Build history of the part. All positions in model axes, mm. Coordinates: 2 decimals unless noted, no trailing zeros. Loops run counter-clockwise (first coordinate to the right, second up) from the corner with the lowest first, then second, coordinate; pieces in that order, holes last.
Item 1: Cut at B-B (z = -2). List the corners of the cut face in (x, y).
Item 2: Cut at A-A (y = -52). List the corners of the cut face in (x, z), and give its area (3 significant figures).
Item 3: Drill centre lines: line 1 along Z through (x, y) = (-51.5, -38); line 2 along Y through (x, z) = (-58, 82); line 3 along Y through (x, z) = (-23, 8.5). Where is each one in solid material? Low to high.
Item 4: Flat gauge pins, fed straight in: pin 1 (2 mm diameter, centred on y = 3.5, z = 7.5, fed in from -X); pin 2 (3 mm diameter, centred on y = -52.5, z = 8, fed in from +X); pin 3 (2 mm diameter, centred on y = -4.5, z = 4.5, fed in from -X). Where does each tip first touch, or does it go through?
from build123d import *

# Parameters (mm, degrees)
BOSS_EXTRU_1_DEPTH = 15
ESQUISSE3_W        = 15
ESQUISSE3_H        = 4
BOSS_EXTRU_2_DEPTH = 2
ESQUISSE4_W        = 15
ESQUISSE4_H        = 12
BOSS_EXTRU_3_DEPTH = 3
BOSS_EXTRU_4_DEPTH = 15
ESQUISSE6_W        = 6
ESQUISSE6_H        = 15
BOSS_EXTRU_5_DEPTH = 15
BOSS_EXTRU_6_DEPTH = 15
ESQUISSE8_W        = 200
ESQUISSE8_H        = 10.22
BOSS_EXTRU_7_DEPTH = 6


with BuildPart() as part:
    # Esquisse1 → Boss.-Extru.1 (new body)
    with BuildSketch(Plane.XY):
        Polygon((0, 4.759390863), (4.68, 1.359390863), (4.68, -3.840609137), (0, -7.240609137), align=None)
    extrude(amount=BOSS_EXTRU_1_DEPTH)

    # Esquisse3 → Boss.-Extru.2 (add)
    with BuildSketch(Plane.ZY):
        with Locations((7.5, -1.240609137)):
            Rectangle(ESQUISSE3_W, ESQUISSE3_H)
    extrude(amount=BOSS_EXTRU_2_DEPTH)

    # Esquisse4 → Boss.-Extru.3 (add)
    with BuildSketch(Plane.ZY.offset(2)):
        with Locations((7.5, -1.240609137)):
            Rectangle(ESQUISSE4_W, ESQUISSE4_H)
    extrude(amount=BOSS_EXTRU_3_DEPTH)

    # Esquisse5 → Boss.-Extru.4 (add)
    with BuildSketch(Plane(origin=(0, 0, 0), x_dir=(-1, 0, 0), z_dir=(0, 0, -1))):
        Polygon((5, 4.759390863), (62.453333234, -43.449679864), (50.453333234, -43.449679864), (5, -7.240609137), align=None)
    extrude(amount=-BOSS_EXTRU_4_DEPTH)

    # Esquisse6 → Boss.-Extru.5 (add)
    with BuildSketch(Plane(origin=(0, -43.449679864, 0), x_dir=(-1, 0, 0), z_dir=(0, -1, 0))):
        with Locations((59.453333234, -7.5)):
            Rectangle(ESQUISSE6_W, ESQUISSE6_H)
    extrude(amount=BOSS_EXTRU_5_DEPTH)

    # Esquisse7 → Boss.-Extru.6 (add)
    with BuildSketch(Plane(origin=(0, 0, 0), x_dir=(-1, 0, 0), z_dir=(0, 0, -1))):
        Polygon((50.453333234, -43.449679864), (56.453333234, -48.229404669), (56.453333234, -43.449679864), align=None)
    extrude(amount=-BOSS_EXTRU_6_DEPTH)

    # Esquisse8 → Boss.-Extru.7 (add)
    with BuildSketch(Plane.ZY.offset(62.453333234)):
        with Locations((7.5, -53.339679864)):
            Rectangle(ESQUISSE8_W, ESQUISSE8_H)
    extrude(amount=-BOSS_EXTRU_7_DEPTH)


solid = part.part
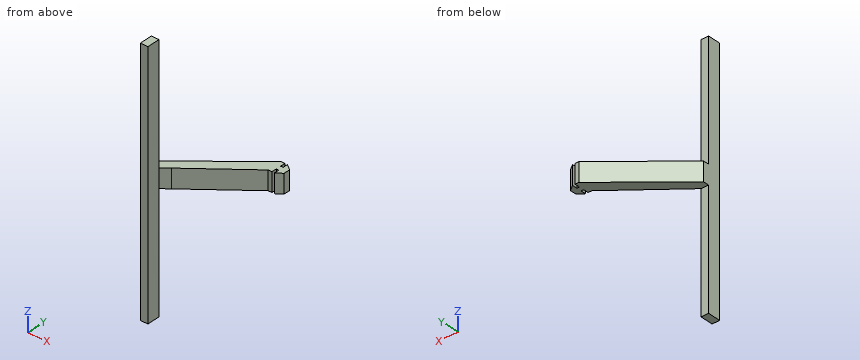
Filled sheet:
1. outline: (-62.45, -58.45) - (-56.45, -58.45) - (-56.45, -48.23) - (-62.45, -48.23) - close
2. outline: (-62.45, -92.5) - (-56.45, -92.5) - (-56.45, 107.5) - (-62.45, 107.5) - close
2. area: 1,200 mm2
3. line 1: z = 0 to 15
3. line 2: y = -58.45 to -48.23
3. line 3: y = -21.58 to -10.34
4. pin 1: stops at x = -7.69
4. pin 2: stops at x = -56.45
4. pin 3: stops at x = -17.23
